For this review, take the finished solid that the model builds, in its own axes (mm). Face numbers are marked on the shaded views. A direction names the side the tool comes from. Coordinates: 2 decimals unless noted, no trailing zeros. Loops run counter-clockwise (first coordinate to the right, second up) from the corner with the lowest first, then second, coordinate; pieces in that order, holes last. Notation, with made-up numbers: M -21,-27.75 L 20,-27.75 A19 cw 20,9.25 Z; hole C 85.5,-17.75 d7. An arc over 180 degrees is marked long. Put each result on its own line as item: value.
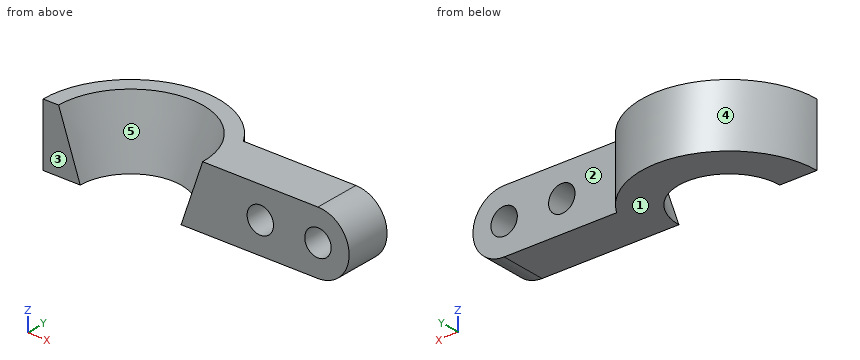
```python
from build123d import *

# Parameters (mm, degrees)
F1_ANGLE = 180
F3_DEPTH = 38
F4_R     = 11
F5_DEPTH = 117


with BuildPart() as f1:
    # F0 (on Front) → F1 (revolve)
    with BuildSketch(Plane.XZ):
        Polygon((-60, 52), (-73, 52), (-73, 0), (-42, 0), align=None)
    revolve(axis=Axis((0, 0, 37.335005), (0, 0, -1)), revolution_arc=F1_ANGLE)

    # F2 (on Front) → F3 (join)
    with BuildSketch(Plane.XZ):
        with BuildLine():
            ThreePointArc((156, 0), (182, 26), (156, 52))
            Line((156, 52), (60, 52))
            Line((60, 52), (42, 0))
            Line((42, 0), (156, 0))
        make_face()
    extrude(amount=-F3_DEPTH)

    # F4 (on face) → F5 (cut)
    with BuildSketch(Plane.XZ):
        with Locations((156, 26)):
            Circle(F4_R)
        with Locations((108, 26)):
            Circle(F4_R)
    extrude(amount=-F5_DEPTH, mode=Mode.SUBTRACT)


solid = f1.part
```
(1) Wall thickness on line 1 along X through (y, z) = (10.5, 29); line 2 along Y through (x, z) = (151, 15); line 3 along X through (y, z) = (36.5, 39.5): over which ranges is each line inside the solid? List them lowest first. Write a range as [from, to].
Determined:
line 1: x = [-72.24, -50.97], [50.97, 97.42], [118.58, 145.42], [166.58, 181.83]
line 2: y = [0, 38]
line 3: x = [-63.22, -42.04], [42.04, 178.22]
(2) Add section D-D (x = 0). Write out the cut boundary in (y, z), plus the area to 3 significant figures.
Determined:
outline: M 42,0 L 73,0 L 73,52 L 60,52 Z
area: 1,140 mm^2
(3) Tool access review of the marked faces 1 and 2: name each direction out of +Z, -Z, +X, -X, +Y, -Y from which nothing blocks a thin tool from reaching the whole face with its end or side.
Determined:
face 1: -Z, +X, -X, +Y, -Y
face 2: +Z, -Z, +X, +Y
(4) Add section A-A (z = 26). Write out the cut boundary in (x, y), plus the area to 3 significant figures.
Determined:
outline: M -73,0 L -51,0 A51 cw 51,0 L 97,0 L 97,38 L 62.33,38 A73 ccw Z; M 119,0 L 145,0 L 145,38 L 119,38 Z; M 167,0 L 182,0 L 182,38 L 167,38 Z
area: 6,890 mm^2
(5) Add section C-C (y = 30.5). State how many separate pieces and enclosed holes the cut face has, plus the area to 3 significant figures.
Determined:
separate pieces: 2
enclosed holes: 2
area: 7,630 mm^2
(6) For pin 1 (1.5 mm diameter, centred on y = 39.5, z = 32, fed in from +X); pin 2 (2 mm diameter, centred on x = 18, z = 36.5, fed in from -Y); pin 3 (12 mm diameter, centred on y = 35, z = 6, fed in from -X), all flat-tipped, find the tip position at first contact; note any pin that passes through.
Determined:
pin 1: stops at x = 61.87
pin 2: stops at y = 51.07
pin 3: stops at x = -66.99
(7) Draft analysis for pull direction X (two halves, no side actions). For the marked faces 3, 4 and 5, state which applies: +X half, -X half, draft (parallel to the pull), parting line (faces both ways), or undercut.
Determined:
face 3: draft
face 4: parting line
face 5: undercut
(8) Add section B-B (x = 108). Write out the cut boundary in (y, z), plus the area to 3 significant figures.
Determined:
outline: M 0,0 L 38,0 L 38,15 L 0,15 Z; M 0,37 L 38,37 L 38,52 L 0,52 Z
area: 1,140 mm^2
